Study the drawing (mm; zero at the part's minimum x, y, z) and answer. A direction names the side the tool comes from. Coordinates: 2 decimals unless noted, no trailing zeros. Loops run counter-clockwise (first coordinate to the right, second up) from the corner with the lowest first, then second, coordinate; pieces in that order, holes last.
Q1. Which of the six approach directions +Z, -Z, +X, -X, +Y, -Y give full straight-line access (tool end or side, diameter ignored) to the marked faces 1, 2 and 3?
Q2. Straight lines are drawn through the part: line 1 (X direction, y = 17.5, z = 12) (3 decimals); line 2 (X direction, y = 4.75, z = 5); line 3 (Z direction, x = 30, y = 20.75). For each, find the intervals that lie inside material, in ascending order.
Q3. Flat-ended cylindrical pins translate along their axes: P1, Ø8, axis at x = 6.5, y = 18, coming from the +Z side; P2, Ø9, axis at x = 30, z = 8, coming from the -Y side; P3, Ø9, axis at x = 7, y = 19, coming from the +Z side; P4, Ø7.5, axis at x = 27, y = 17, coming from the -Z side. Find the tip coordinate at first contact, or state that the pin passes through.
Q4. Section C-C (z = 8) is taken. Give the vertices of the cut face in (x, y) (3 decimals).
Q5. Section A-A (x = 51.5) is taken. Give the vertices of the cut face in (y, z).
Q6. Section D-D (x = 30) is taken. Give the vertices of the cut face in (y, z), then the cut area to 3 significant figures.
Q7. The mould has two halves that part along Z. Classify the marked faces 4, 5, 6 and 7: pulls with the +Z half, pulls with the -Z half, needs draft (parallel to the pull), parting line crosses it, or undercut.
Q8. Section B-B (y = 12.5) is taken. Give the vertices of the cut face in (x, z), then the cut area to 3 significant figures.
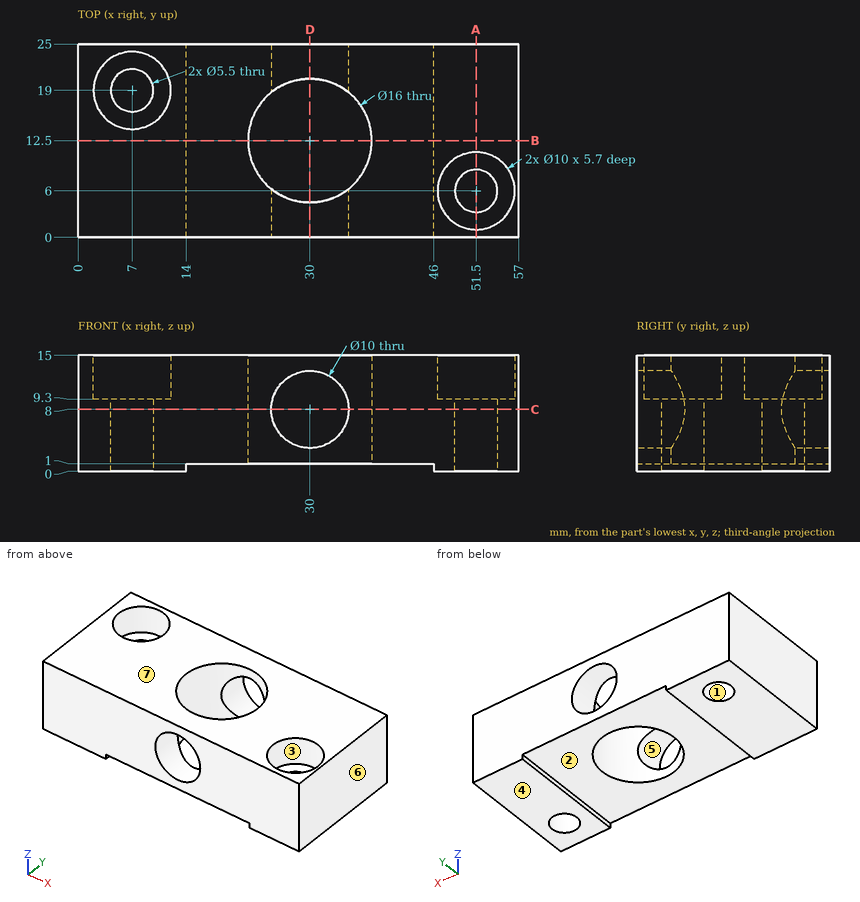
Numbers:
1. face 1: +Z, -Z
1. face 2: -Z, +Y, -Y
1. face 3: +Z
2. line 1: x = 0 to 2.23, 11.77 to 23.755, 36.245 to 57
2. line 2: x = 0 to 26, 34 to 49.05, 53.95 to 57
2. line 3: z = 1 to 3, 13 to 15
3. P1: stops at z = 15
3. P2: passes through
3. P3: stops at z = 9.3
3. P4: stops at z = 1
4. outline: (0, 0) - (25, 0) - (25, 6.255) arc R8 cw to (25, 18.745) - (25, 25) - (0, 25) - close; (35, 0) - (57, 0) - (57, 25) - (35, 25) - (35, 18.745) arc R8 cw to (35, 6.255) - close; hole circle Ø5.5 at (7, 19); hole circle Ø5.5 at (51.5, 6)
5. outline: (0, 0) - (3.25, 0) - (3.25, 9.3) - (1, 9.3) - (1, 15) - (0, 15) - close; (8.75, 0) - (25, 0) - (25, 15) - (11, 15) - (11, 9.3) - (8.75, 9.3) - close
6. outline: (0, 1) - (4.5, 1) - (4.5, 3) - (0, 3) - close; (0, 13) - (4.5, 13) - (4.5, 15) - (0, 15) - close; (20.5, 1) - (25, 1) - (25, 3) - (20.5, 3) - close; (20.5, 13) - (25, 13) - (25, 15) - (20.5, 15) - close
6. area: 36.0 mm2
7. face 4: pulls with the -Z half
7. face 5: undercut
7. face 6: needs draft
7. face 7: pulls with the +Z half
8. outline: (0, 0) - (14, 0) - (14, 1) - (22, 1) - (22, 15) - (0, 15) - close; (38, 1) - (46, 1) - (46, 0) - (57, 0) - (57, 15) - (38, 15) - close
8. area: 599 mm2
